Can you work these out from the drawing? Everything is in mm from the part's minimum corner. A direction names the side the tool comes from. Round coordinates to 2 decimals unless told otherwise and drop trailing zeros. Order: outer loops, then holes, each group sorted by start corner. A loop starts at its lowest first (then second) coordinate and runs counter-clockwise, first axis right, second up. Notation, with made-up numbers: M -15.5,32.5 L -3.5,32.5 A9 cw -3.5,47.5 Z; hole C -5.5,-23 d10. An arc over 180 degrees is marked long. Write item = value, one per line. Start each with the question number.
Item 1: I want a section at D-D, the plane x = 2. List the corners of the cut face in (y, z) for me.
Item 2: I want a section at C-C, the plane y = 2.25. List the corners of the cut face in (x, z) for me.
Item 3: I want a section at A-A, the plane x = 3.81. List the corners of the cut face in (y, z) for me (1 decimal).
Item 4: We'd pull the mould along X, two halves only. Please class the marked faces 1, 2 and 3: pulls with the +X half, pulls with the -X half, needs draft (parallel to the pull), parting line crosses it, or undercut.
Item 5: I want a section at B-B, the plane z = 1.15. List the corners of the cut face in (x, y) for me (1 decimal).
Item 6: I'm going to push a flat-ended pin straight in: P1, Ø1, axis at x = 6.5, y = 1, coming from the +Z side. Where does the tip first touch, or does it pass through?
Item 7: Please list where these lines run through material, in increasing order: L1, parallel to Y at x = 3.81, z = 0.7 (1 decimal); L2, parallel to X at y = 4.25, z = 1.1; L3, parallel to X at y = 4.5, z = 1.05.
Item 8: For the marked faces 4 and 5, which set-ups out of +Z, -Z, +X, -X, +Y, -Y let a thin tool reach every point of the face, with its end or its side?
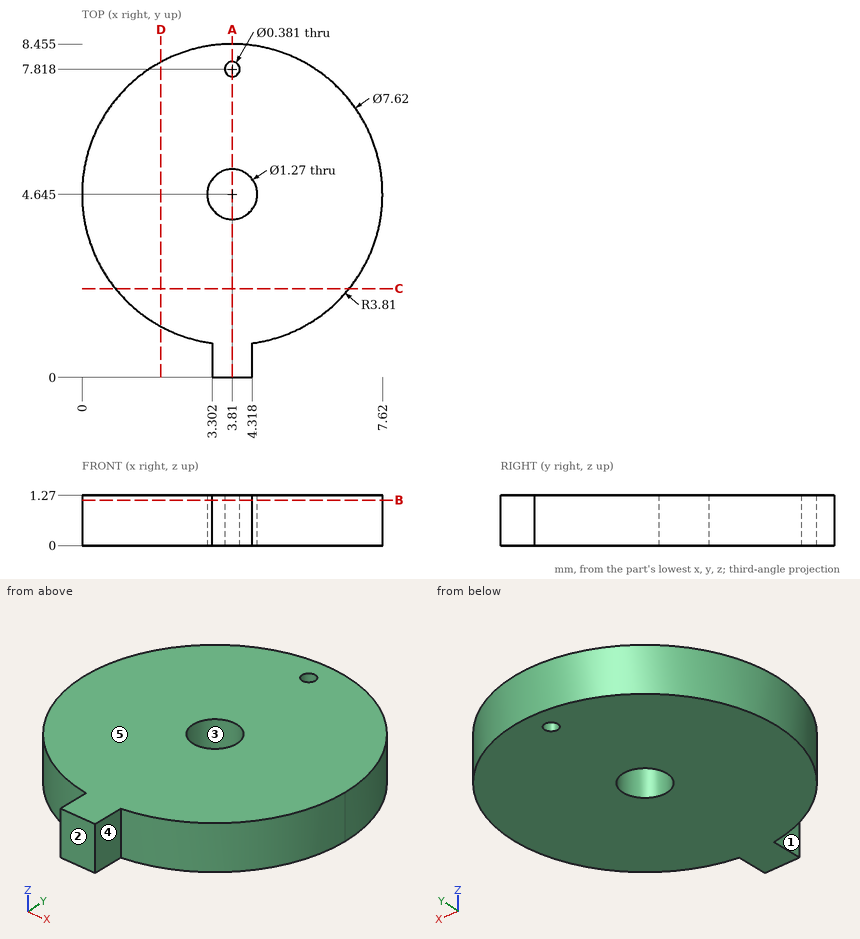
Filled in:
q1.outline = M 1.29,0 L 8,0 L 8,1.27 L 1.29,1.27 Z
q2.outline = M 0.85,0 L 6.77,0 L 6.77,1.27 L 0.85,1.27 Z
q3.outline = M 0,0 L 4,0 L 4,1.3 L 0,1.3 Z; M 5.3,0 L 7.6,0 L 7.6,1.3 L 5.3,1.3 Z; M 8,0 L 8.5,0 L 8.5,1.3 L 8,1.3 Z
q4.face_1 = pulls with the -X half
q4.face_2 = needs draft
q4.face_3 = undercut
q5.outline = M 3.3,0 L 4.3,0 L 4.3,0.9 A3.8 ccw long 3.3,0.9 Z; hole C 3.8,4.6 d1.3; hole C 3.8,7.8 d0.4
q6.P1 = through
q7.L1 = 0 to 4, 5.3 to 7.6, 8 to 8.5
q7.L2 = 0.02 to 3.31, 4.31 to 7.6
q7.L3 = 0 to 3.19, 4.43 to 7.62
q8.face_4 = +Z, -Z, +X, -Y
q8.face_5 = +Z, +X, -X, +Y, -Y
